```python
from build123d import *

# Parameters (mm, degrees)
SKETCH2_R                       = 48.5
SKETCH2_R_2                     = 1.5
BOSS_EXTRUDE1_DEPTH             = 4
SKETCH3_R                       = 3.75
CUT_EXTRUDE1_DEPTH              = 1.5
BOSS_EXTRUDE2_START             = 4
SKETCH4_R                       = 9
BOSS_EXTRUDE2_DEPTH             = 14
CUT_EXTRUDE2_START              = 6
SKETCH6_R                       = 1.325
CUT_EXTRUDE2_DEPTH              = 93.806192047
BOSS_EXTRUDE3_DEPTH             = 9
BOSS_EXTRUDE3_DIRECTION_2_REACH = 110.778
CUT_EXTRUDE3_DEPTH              = 105.285680763
FILLET1_R                       = 10
FILLET2_R                       = 2


with BuildPart() as part:
    # Sketch2 → Boss-Extrude1 (new body)
    with BuildSketch(Plane(origin=(0, 0, 0), x_dir=(1, 0, 0), z_dir=(0, 1, 0))):
        with Locations(Location((0, 0, 0), (0, 0, 270))):
            Circle(SKETCH2_R)
        with Locations(Location((0, 7.25, 0), (0, 0, 270))):
            Circle(SKETCH2_R_2, mode=Mode.SUBTRACT)
        with Locations(Location((0, -7.25, 0), (0, 0, 270))):
            Circle(SKETCH2_R_2, mode=Mode.SUBTRACT)
    extrude(amount=-BOSS_EXTRUDE1_DEPTH)

    # Sketch3 → Cut-Extrude1 (cut)
    with BuildSketch(Plane(origin=(0, -4, 0), x_dir=(-1, 0, 0), z_dir=(0, -1, 0))):
        with Locations(Location((0, 0, 0), (0, 0, 90))):
            Circle(SKETCH3_R)
    extrude(amount=-CUT_EXTRUDE1_DEPTH, mode=Mode.SUBTRACT)

    # Sketch4 → Boss-Extrude2 (add)
    with BuildSketch(Plane(origin=(0, 0, 0), x_dir=(0, 0, -1), z_dir=(1, 0, 0)).offset(BOSS_EXTRUDE2_START)):
        with BuildLine():
            Line((-14.470153899, 52.351446146), (-27.529193782, 21.649444314))
            ThreePointArc((-27.529193782, 21.649444314), (-29.630146994, 14.89650137), (-30.34, 7.86))
            Line((-30.34, 7.86), (-30.34, 0))
            Line((-30.34, 0), (31.097052925, 0))
            Line((31.097052925, 0), (31.097052925, 7.64))
            ThreePointArc((31.097052925, 7.64), (32.258997722, 13.428629218), (35.564816687, 18.320449421))
            ThreePointArc((35.564816687, 18.320449421), (31.254587763, 65.781337665), (-14.470153899, 52.351446146))
        make_face()
        with Locations((13.91, 40.28)):
            Circle(SKETCH4_R, mode=Mode.SUBTRACT)
    extrude(amount=BOSS_EXTRUDE2_DEPTH)

    # Sketch6 → Cut-Extrude2 (cut, through all)
    with BuildSketch(Plane(origin=(0, 0, 0), x_dir=(0, 0, -1), z_dir=(1, 0, 0)).offset(CUT_EXTRUDE2_START)):
        with Locations(Location((20.674280786, 54.114591003, 0), (0, 0, 180))):
            Circle(SKETCH6_R)
        with Locations(Location((27.745348598, 47.043523191, 0), (0, 0, 180))):
            Circle(SKETCH6_R)
        with Locations(Location((-7.352145163, 11.94602943, 0), (0, 0, 180))):
            Circle(SKETCH6_R)
        with Locations(Location((-14.423212974, 19.017097242, 0), (0, 0, 180))):
            Circle(SKETCH6_R)
        Polygon((-0.41, 11.11), (-15.259242405, 25.959242405), (13.732135624, 54.950620434), (28.581378029, 40.101378029), align=None)
    extrude(amount=CUT_EXTRUDE2_DEPTH, mode=Mode.SUBTRACT)

    # Sketch8 → Boss-Extrude3 (add)
    with BuildSketch(Plane(origin=(18, 0, 0), x_dir=(0, 0, -1), z_dir=(1, 0, 0))):
        with BuildLine():
            Line((37.097052925, 0), (37.097052925, 7.64))
            ThreePointArc((37.097052925, 7.64), (37.794219803, 11.113177531), (39.777711182, 14.048269653))
            ThreePointArc((39.777711182, 14.048269653), (34.628937191, 70.742563919), (-19.991447191, 54.69991807))
            Line((-19.991447191, 54.69991807), (-33.050487075, 23.997916239))
            ThreePointArc((-33.050487075, 23.997916239), (-35.509252358, 16.094883664), (-36.34, 7.86))
            Line((-36.34, 7.86), (-36.34, 0))
            Line((-36.34, 0), (-27.34, 0))
            ThreePointArc((-27.34, 0), (-23.018237165, 26.695212958), (-14.470153899, 52.351446146))
            ThreePointArc((-14.470153899, 52.351446146), (31.254587763, 65.781337665), (35.564816687, 18.320449421))
            ThreePointArc((35.564816687, 18.320449421), (32.258997722, 13.428629218), (31.097052925, 7.64))
            Line((31.097052925, 7.64), (31.097052925, 0))
            Line((31.097052925, 0), (37.097052925, 0))
        make_face()
    extrude(amount=BOSS_EXTRUDE3_DEPTH)

    # Boss-Extrude3 direction 2: up to this face of the body (flat: up to its plane)
    boss_extrude3_direction_2_end = Plane(part.part.faces().sort_by_distance((4, 32.037892767, -8.057594293))[0])
    # Sketch8 → Boss-Extrude3 direction 2 (add, up to the picked face)
    with BuildSketch(Plane(origin=(18, 0, 0), x_dir=(0, 0, -1), z_dir=(1, 0, 0)), mode=Mode.PRIVATE) as boss_extrude3_direction_2_sk1:
        with BuildLine():
            Line((37.097052925, 0), (37.097052925, 7.64))
            ThreePointArc((37.097052925, 7.64), (37.794219803, 11.113177531), (39.777711182, 14.048269653))
            ThreePointArc((39.777711182, 14.048269653), (34.628937191, 70.742563919), (-19.991447191, 54.69991807))
            Line((-19.991447191, 54.69991807), (-33.050487075, 23.997916239))
            ThreePointArc((-33.050487075, 23.997916239), (-35.509252358, 16.094883664), (-36.34, 7.86))
            Line((-36.34, 7.86), (-36.34, 0))
            Line((-36.34, 0), (-27.34, 0))
            ThreePointArc((-27.34, 0), (-23.018237165, 26.695212958), (-14.470153899, 52.351446146))
            ThreePointArc((-14.470153899, 52.351446146), (31.254587763, 65.781337665), (35.564816687, 18.320449421))
            ThreePointArc((35.564816687, 18.320449421), (32.258997722, 13.428629218), (31.097052925, 7.64))
            Line((31.097052925, 7.64), (31.097052925, 0))
            Line((31.097052925, 0), (37.097052925, 0))
        make_face()
    boss_extrude3_direction_2_tool1 = split(extrude(boss_extrude3_direction_2_sk1.sketch, amount=-BOSS_EXTRUDE3_DIRECTION_2_REACH, mode=Mode.PRIVATE), bisect_by=boss_extrude3_direction_2_end, keep=Keep.BOTH, mode=Mode.PRIVATE)
    add(boss_extrude3_direction_2_tool1.solids().sort_by(Axis((18, 66.743228, -31.908812), (-1, 0, 0)))[0])

    # Sketch9 → Cut-Extrude3 (cut, through all)
    with BuildSketch(Plane.XY):
        with BuildLine():
            Line((27, 77.12076762), (21, 77.12076762))
            ThreePointArc((21, 77.12076762), (22.257085893, 38.453914076), (26.5, 0))
            Line((26.5, 0), (27, 0))
            Line((27, 0), (27, 77.12076762))
        make_face()
    extrude(amount=-CUT_EXTRUDE3_DEPTH, mode=Mode.SUBTRACT)

    # Fillet1
    fillet1_edges = [part.edges().sort_by_distance(p)[0] for p in [
        (4, 3.82, -37.097052925),
        (4, 11.113177531, -37.794219803),
        (4, 70.742563919, -34.628937191),
        (4, 39.348917154, 26.520967133),
        (4, 16.094883664, 35.509252358),
        (4, 3.93, 36.34),
    ]]
    fillet(fillet1_edges, radius=FILLET1_R)

    # Fillet2
    fillet2_edges = [part.edges().sort_by_distance(p)[0] for p in [
        (20.25, 0, -37.097052925),
        (4, 0, -0.378526462),
        (20.5, 0, 36.34),
        (6.928932188, 0, -34.168120736),
        (6.928932188, 0, 33.411067812),
    ]]
    fillet(fillet2_edges, radius=FILLET2_R)


solid = part.part
```
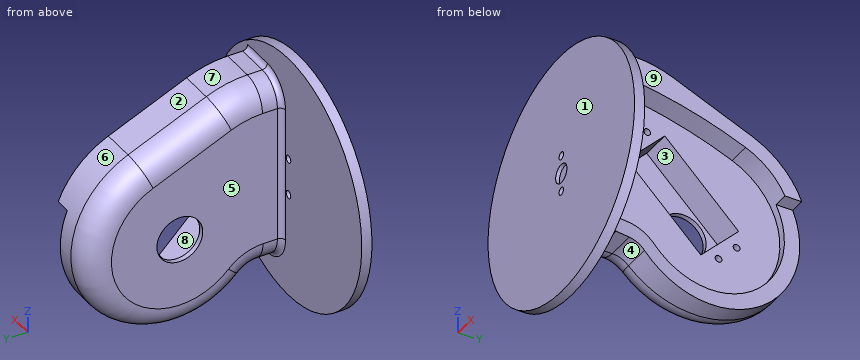
The model under review builds one solid part; all positions refer to its coordinate system, in mm. Face numbers are marked on the shaded views. A direction names the side the tool comes from. Coordinates: 2 decimals unless noted, no trailing zeros. Write each loop counter-clockwise with the first axis right and the second up, starting at its lowest first coordinate (ties: lowest second). Pieces come first, ordered by that corner, then holes.
1) We need section B-B on z = -7.25. Count the separate pieces of the cut face and the enclosed holes in it, then the cut area to 3 significant figures.
2) Machinability: for the marked faces 5, 6, 7, 8 and 9, which of the approach directions +Z, -Z, +X, -X, +Y, -Y give a long, thin tool a straight path to every point of the face, cutting with its end or side? Answer none if there is none.
3) Clearance check with flat-ended pins moving along their axes: pin 1 Ø3 at (x, y) = (23, 5) entering from -Z; pin 2 Ø2.5 at (y, z) = (54.11, -20.67) entering from -X; pin 3 Ø3 at (y, z) = (11.5, 7.5) entering from +X. State where each tip first meets the part, or that it passes through.
4) The part is to be moulded in two halves that separate along Z. For the marked faces 1, 2, 3 and 4, say which applies: pulls with the +Z half, pulls with the -Z half, needs draft (parallel to the pull), parting line crosses it, or undercut.
5) We need section D-D on x = 37. State the section outline as (y, z) points.
6) We need section C-C on x = -35. State the section outline as (y, z) points, then the cut area to 3 significant figures.
7) To check wall thickness, follow probe 1 along Y at (x, z) = (0, 25); probe 2 along X at (y, z) = (8, 23); probe 3 along Y at (x, z) = (23, 1.5). State the ranges of each line that lie inside material, in increasing order.
8) We need section A-A on x = 0. State the section outline as (y, z) points.
Answer list:
1. separate pieces: 3
1. enclosed holes: 0
1. area: 1,060 mm2
2. face 5: +Z, -Z, -X, +Y
2. face 6: +X, -X
2. face 7: +Z, +X, -X, +Y
2. face 8: +X
2. face 9: +Z, -Z, +X, +Y
3. pin 1: stops at z = -37.1
3. pin 2: stops at x = 4
3. pin 3: stops at x = 18
4. face 1: needs draft
4. face 2: pulls with the +Z half
4. face 3: undercut
4. face 4: pulls with the -Z half
5. outline: (-4, -31.36) - (0, -31.36) - (0, 31.36) - (-4, 31.36) - close
6. outline: (-4, -33.57) - (0, -33.57) - (0, 33.57) - (-4, 33.57) - close
6. area: 269 mm2
7. probe 1: y = -4 to 0
7. probe 2: x = 4 to 18
7. probe 3: y = -4 to 0, 66.99 to 73.74
8. outline: (-4, -48.5) - (0, -48.5) - (0, -8.75) - (-4, -8.75) - close; (-4, -5.75) - (0, -5.75) - (0, 5.75) - (-4, 5.75) - (-4, 3.75) - (-2.5, 3.75) - (-2.5, -3.75) - (-4, -3.75) - close; (-4, 8.75) - (0, 8.75) - (0, 48.5) - (-4, 48.5) - close
